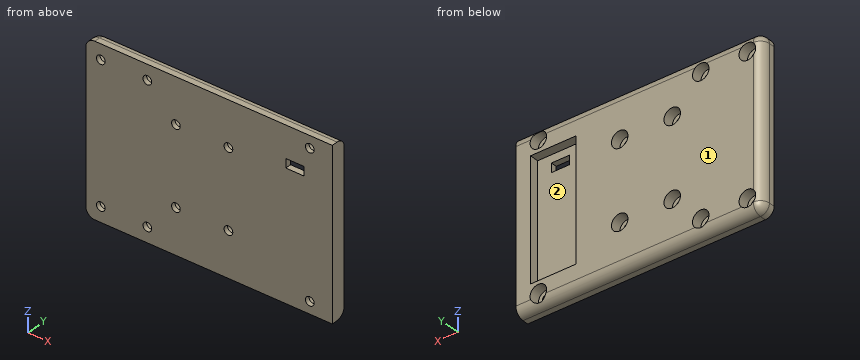
from build123d import *

# Parameters (mm, degrees)
SKETCH1_W                        = 82.1
SKETCH1_H                        = 56
BOSS_EXTRUDE1_DEPTH              = 5
CBORE_FOR_M2_5_SHCS1_D           = 2.9
CBORE_FOR_M2_5_SHCS1_CBORE_D     = 5.5
CBORE_FOR_M2_5_SHCS1_CBORE_DEPTH = 3.5
FILLET1_R                        = 3
FILLET2_R                        = 3
SKETCH4_W                        = 15
SKETCH4_H                        = 40
CUT_EXTRUDE1_DEPTH               = 3
SKETCH5_W                        = 6
SKETCH5_H                        = 3
CUT_EXTRUDE2_DEPTH               = 50.780543533
MOVE_FACE1_BY                    = 0.1
MOVE_FACE1_2_BY                  = 0.1
MOVE_FACE1_3_BY                  = 0.1
MOVE_FACE1_4_BY                  = 0.1


with BuildPart() as part:
    # Sketch1 → Boss-Extrude1 (new body)
    with BuildSketch(Plane(origin=(0, 0, 0), x_dir=(1, 0, 0), z_dir=(0, 1, 0))):
        Rectangle(SKETCH1_W, SKETCH1_H)
    extrude(amount=BOSS_EXTRUDE1_DEPTH)

    # CBORE for M2.5 SHCS1 (through all)
    with Locations(Plane(origin=(0, 5, 0), x_dir=(1, 0, 0), z_dir=(0, 1, 0))):
        with Locations((-36.05, 23), (-36.05, -23), (-20.55, -23), (-20.55, 23), (-11.05, -13), (-11.05, 13), (6.45, 13), (6.45, -13), (33.55, 24), (33.55, -24)):
            CounterBoreHole(CBORE_FOR_M2_5_SHCS1_D / 2, CBORE_FOR_M2_5_SHCS1_CBORE_D / 2, CBORE_FOR_M2_5_SHCS1_CBORE_DEPTH)

    # Fillet1
    fillet1_edges = [part.edges().sort_by_distance(p)[0] for p in [
        (-41.05, 2.5, 28),
        (-41.05, 2.5, -28),
    ]]
    fillet(fillet1_edges, radius=FILLET1_R)

    # Fillet2
    # the kernel refuses this fillet: 3 mm, written as the material it takes off along each edge
    with BuildSketch(Plane(origin=(-38.05, 5, 28), x_dir=(0, -1, 0), z_dir=(1, 0, 0))) as fillet2_piece_1:
        with BuildLine():
            CenterArc((FILLET2_R, FILLET2_R), FILLET2_R, 180, 90)
            Line((0, FILLET2_R), (0, 0))
            Line((0, 0), (FILLET2_R, 0))
        make_face()
    extrude(amount=86.6, mode=Mode.SUBTRACT)
    with BuildSketch(Plane(origin=(-38.05, 5, 25), x_dir=(0, 0, 1), z_dir=(1, 0, 0))) as fillet2_piece_2:
        with BuildLine():
            CenterArc((3 - FILLET2_R, FILLET2_R), FILLET2_R, 270, 90)
            Line((3 - FILLET2_R, 0), (3, 0))
            Line((3, 0), (3, FILLET2_R))
        make_face()
    revolve(axis=Axis((-38.05, 5, 25), (0, -1, 0)), revolution_arc=90, mode=Mode.SUBTRACT)
    with BuildSketch(Plane(origin=(-38.05, 5, -25), x_dir=(-1, 0, 0), z_dir=(0, 0, 1))) as fillet2_piece_3:
        with BuildLine():
            CenterArc((3 - FILLET2_R, FILLET2_R), FILLET2_R, 270, 90)
            Line((3, FILLET2_R), (3, 0))
            Line((3, 0), (3 - FILLET2_R, 0))
        make_face()
    revolve(axis=Axis((-38.05, 5, -25), (0, -1, 0)), revolution_arc=90, mode=Mode.SUBTRACT)
    with BuildSketch(Plane(origin=(48.55, 5, -28), x_dir=(0, 0, 1), z_dir=(-1, 0, 0))) as fillet2_piece_4:
        with BuildLine():
            CenterArc((FILLET2_R, -FILLET2_R), FILLET2_R, 90, 90)
            Line((0, -FILLET2_R), (0, 0))
            Line((0, 0), (FILLET2_R, 0))
        make_face()
    extrude(amount=86.6, mode=Mode.SUBTRACT)
    with BuildSketch(Plane(origin=(-41.05, 5, -25), x_dir=(1, 0, 0), z_dir=(0, 0, 1))) as fillet2_piece_5:
        with BuildLine():
            CenterArc((FILLET2_R, -FILLET2_R), FILLET2_R, 90, 90)
            Line((0, -FILLET2_R), (0, 0))
            Line((0, 0), (FILLET2_R, 0))
        make_face()
    extrude(amount=50, mode=Mode.SUBTRACT)

    # Sketch4 → Cut-Extrude1 (cut)
    with BuildSketch(Plane(origin=(0, 5, 0), x_dir=(1, 0, 0), z_dir=(0, 1, 0))):
        with Locations((28.55, 0)):
            Rectangle(SKETCH4_W, SKETCH4_H)
    extrude(amount=-CUT_EXTRUDE1_DEPTH, mode=Mode.SUBTRACT)

    # Sketch5 → Cut-Extrude2 (cut, through all)
    with BuildSketch(Plane(origin=(0, 2, 0), x_dir=(1, 0, 0), z_dir=(0, 1, 0))):
        with Locations((28.55, -16)):
            Rectangle(SKETCH5_W, SKETCH5_H)
    extrude(amount=-CUT_EXTRUDE2_DEPTH, mode=Mode.SUBTRACT)

    # Move Face1: a face moved inward by 0.1
    extrude(part.faces().sort_by_distance((28.55, 3.5, 20))[0], amount=MOVE_FACE1_BY, dir=(0, 0, 1), mode=Mode.SUBTRACT)

    # Move Face1 2: a face moved inward by 0.1
    extrude(part.faces().sort_by_distance((36.05, 3.5, 0))[0], amount=MOVE_FACE1_2_BY, dir=(1, 0, 0), mode=Mode.SUBTRACT)

    # Move Face1 3: a face moved inward by 0.1
    extrude(part.faces().sort_by_distance((28.55, 3.5, -20))[0], amount=MOVE_FACE1_3_BY, dir=(0, 0, -1), mode=Mode.SUBTRACT)

    # Move Face1 4: a face moved inward by 0.1
    extrude(part.faces().sort_by_distance((21.05, 3.5, 0))[0], amount=MOVE_FACE1_4_BY, dir=(-1, 0, 0), mode=Mode.SUBTRACT)


solid = part.part
Design review of the part built by this model. Coordinates are the model's own, in mm. Face numbers are marked on the shaded views. Round coordinates to 2 decimals unless told otherwise and drop trailing zeros. Write each loop counter-clockwise with the first axis right and the second up, starting at its lowest first coordinate (ties: lowest second). Pieces come first, ordered by that corner, then holes. Notation, with made-up numbers: (44, 28) -> (65, 28) arc R18 ccw to (65, 45) -> close; hole circle Ø5 at (-10, -38). An arc over 180 degrees is marked (long way). One line per item, written item: value. Start each with the question number.
Q1. Insertion check: P1, Ø6.5, axis at x = 33.55, z = -24, coming from the +Y side; P2, Ø2.5, axis at x = 6.5, z = -14, coming from the +Y side. Each pin has a flat end and moves straight along its axis. Give the tip position at first contact, or say it passes through.
Q2. To check wall thickness, follow probe 1 along Z at (x, y) = (6.45, 1.05); probe 2 along Z at (x, y) = (33.55, 0.45); probe 3 along X at (y, z) = (1.7, -11). State the ranges of each line that lie inside material, in increasing order.
Q3. Add section D-D (y = 4.2). State how many separate pieces and enclosed holes the cut face has, then the cut area to 3 significant figures.
Q4. Add section A-A (x = -11.05). Give the boundary of the cut face in (y, z).
Q5. Add section B-B (z = 13). Give the boundary of the cut face in (x, y), then the cut area to 3 significant figures.
Q6. Add section C-C (z = -8). Give the boundary of the cut face in (x, y).
Q7. The part is to be moulded in two halves that separate along Z. For the marked faces 1 and 2, say which applies: pulls with the +Z half, pulls with the -Z half, needs draft (parallel to the pull), parting line crosses it, or undercut.
Response:
1. P1: stops at y = 5
1. P2: stops at y = 1.5
2. probe 1: z = -28 to -14.45, -11.55 to 11.55, 14.45 to 28
2. probe 2: z = -28 to -25.45, -22.55 to 22.55, 25.45 to 28
2. probe 3: x = -41.05 to -12.94, -9.16 to 4.56, 8.34 to 41.05
3. separate pieces: 1
3. enclosed holes: 11
3. area: 3,540 mm^2
4. outline: (0, -28) -> (2, -28) arc R3 ccw to (5, -25) -> (5, -15.75) -> (1.5, -15.75) -> (1.5, -14.45) -> (0, -14.45) -> close; (0, -11.55) -> (1.5, -11.55) -> (1.5, -10.25) -> (5, -10.25) -> (5, 10.25) -> (1.5, 10.25) -> (1.5, 11.55) -> (0, 11.55) -> close; (0, 14.45) -> (1.5, 14.45) -> (1.5, 15.75) -> (5, 15.75) -> (5, 25) arc R3 ccw to (2, 28) -> (0, 28) -> close
5. outline: (-41.05, 0) -> (-12.5, 0) -> (-12.5, 1.5) -> (-13.8, 1.5) -> (-13.8, 5) -> (-38.05, 5) arc R3 ccw to (-41.05, 2) -> close; (-9.6, 0) -> (5, 0) -> (5, 1.5) -> (3.7, 1.5) -> (3.7, 5) -> (-8.3, 5) -> (-8.3, 1.5) -> (-9.6, 1.5) -> close; (7.9, 0) -> (41.05, 0) -> (41.05, 5) -> (36.15, 5) -> (36.15, 2) -> (20.95, 2) -> (20.95, 5) -> (9.2, 5) -> (9.2, 1.5) -> (7.9, 1.5) -> close
5. area: 316 mm^2
6. outline: (-41.05, 0) -> (41.05, 0) -> (41.05, 5) -> (36.15, 5) -> (36.15, 2) -> (20.95, 2) -> (20.95, 5) -> (-38.05, 5) arc R3 ccw to (-41.05, 2) -> close
7. face 1: needs draft
7. face 2: undercut
